Can you work these out from the model? Positions are in its coordinate system, mm. A direction names the side the tool comes from. Coordinates: 2 decimals unless noted, no trailing zeros. Order: outer loops, then holes, each group sorted by start corner. A loop starts at its lowest first (then second) coordinate and runs counter-clockwise, first axis right, second up. Notation, with made-up numbers: (-38, 51) -> (-1, 51) arc R20 ccw to (-1, 80) -> close; hole circle Ø2 at (67.5, 53). An arc over 180 degrees is marked (long way). Answer in a Markdown table with one row per item. Add a question column.
1. If I drill on line 1 along Z through (x, y) = (0.7, 23); line 2 along Y through (x, z) = (0.5, -60); line 3 along Y through (x, z) = (0.35, -26), over which ranges is the centre line in solid material (lowest first)? Write a range as [from, to].
2. Will these pins go through, and if not, where does the flat tip stop? pin 1 (1 mm diameter, centred on x = 0.5, z = -107.5, fed in from +Y); pin 2 (1 mm diameter, centred on x = 1.5, z = -105, fed in from -Y); pin 3 (1 mm diameter, centred on x = 1.5, y = 32, fed in from +Z); pin 4 (4 mm diameter, centred on y = 23.5, z = -82.5, fed in from -X).
3. We'd pull the mould along Y, two halves only. Please class faces 4 (the face through (1.01, 25.4, -6.57)), 5 (the face through (1, 16, 5)), 6 (the face through (1, 31, -2)): pulls with the +Y half, pulls with the -Y half, needs draft (parallel to the pull), parting line crosses it, or undercut.
4. Imagine slicing it at A-A on z = -78. Write out the boundary of the cut face in (x, y).
5. Imagine slicing it at D-D on x = 0.4. State how many separate pieces and enclosed holes the cut face has, plus the area to 3 significant figures.
6. Imagine slicing it at C-C on z = -45. Write out the boundary of the cut face in (x, y).
7. On a 3-axis mill with a long thin cutter (end or side, diameter ignored), from which of +Z, -Z, +X, -X, +Y, -Y can I reach the whole of each face in a straight line? I mean faces 1 (the face through (1, 18, 1)), 2 (the face through (1, 32, -82)), 3 (the face through (1, 31, -106)). Say none if no direction works.
8. Imagine slicing it at B-B on y = 6. Write out the boundary of the cut face in (x, z).
from build123d import *

# Parameters (mm, degrees)
SKETCH_1_W          = 107
SKETCH_1_H          = 31
EXTRUDE_1_DEPTH     = 2
EXTRUDE_2_DEPTH     = 2
CUT_EXTRUDE_1_DEPTH = 117.228223767
SKETCH_5_W          = 15
SKETCH_5_H          = 2.5
EXTRUDE_3_DEPTH     = 2
CUT_EXTRUDE_2_DEPTH = 117.919844338
CUT_EXTRUDE_3_DEPTH = 117.919844338


with BuildPart() as part:
    # 草图1 → 凸台-拉伸1 (new body)
    with BuildSketch(Plane(origin=(0, 0, 0), x_dir=(0, 0, -1), z_dir=(1, 0, 0))):
        with Locations((53.5, 15.5)):
            Rectangle(SKETCH_1_W, SKETCH_1_H)
    extrude(amount=EXTRUDE_1_DEPTH)

    # 草图2 → 凸台-拉伸2 (add)
    with BuildSketch(Plane(origin=(2, 0, 0), x_dir=(0, 0, -1), z_dir=(1, 0, 0))):
        Polygon((0, 31), (-5, 31), (-5, 0), (0, 0), (0, 5), (-2.1, 5), (-2.1, 13), (0, 13), (0, 18), (-2.1, 18), (-2.1, 26), (0, 26), align=None)
        Polygon((107, 0), (107, 5), (109.1, 5), (109.1, 13), (107, 13), (107, 18), (109.1, 18), (109.1, 26), (107, 26), (107, 31), (112, 31), (112, 0), align=None)
    extrude(amount=-EXTRUDE_2_DEPTH)

    # 草图3 → 切除-拉伸1 (cut, through all)
    with BuildSketch(Plane(origin=(2, 0, 0), x_dir=(0, 0, -1), z_dir=(1, 0, 0))):
        with BuildLine():
            Line((-2.1, 24), (-2.1, 26))
            ThreePointArc((-2.1, 26), (-3.1, 25), (-2.1, 24))
        make_face()
        with BuildLine():
            Line((0, 24), (0, 26))
            ThreePointArc((0, 26), (1, 25), (0, 24))
        make_face()
        with BuildLine():
            Line((0, 20), (0, 18))
            ThreePointArc((0, 18), (1, 19), (0, 20))
        make_face()
        with BuildLine():
            Line((-2.1, 20), (-2.1, 18))
            ThreePointArc((-2.1, 18), (-3.1, 19), (-2.1, 20))
        make_face()
        with BuildLine():
            Line((-2.1, 11), (-2.1, 13))
            ThreePointArc((-2.1, 13), (-3.1, 12), (-2.1, 11))
        make_face()
        with BuildLine():
            Line((0, 11), (0, 13))
            ThreePointArc((0, 13), (1, 12), (0, 11))
        make_face()
        with BuildLine():
            Line((0, 7), (0, 5))
            ThreePointArc((0, 5), (1, 6), (0, 7))
        make_face()
        with BuildLine():
            Line((-2.1, 7), (-2.1, 5))
            ThreePointArc((-2.1, 5), (-3.1, 6), (-2.1, 7))
        make_face()
        with BuildLine():
            Line((109.1, 7), (109.1, 5))
            ThreePointArc((109.1, 5), (110.1, 6), (109.1, 7))
        make_face()
        with BuildLine():
            Line((107, 7), (107, 5))
            ThreePointArc((107, 5), (106, 6), (107, 7))
        make_face()
        with BuildLine():
            Line((107, 11), (107, 13))
            ThreePointArc((107, 13), (106, 12), (107, 11))
        make_face()
        with BuildLine():
            Line((109.1, 11), (109.1, 13))
            ThreePointArc((109.1, 13), (110.1, 12), (109.1, 11))
        make_face()
        with BuildLine():
            Line((109.1, 20), (109.1, 18))
            ThreePointArc((109.1, 18), (110.1, 19), (109.1, 20))
        make_face()
        with BuildLine():
            Line((107, 20), (107, 18))
            ThreePointArc((107, 18), (106, 19), (107, 20))
        make_face()
        with BuildLine():
            Line((107, 24), (107, 26))
            ThreePointArc((107, 26), (106, 25), (107, 24))
        make_face()
        with BuildLine():
            Line((109.1, 24), (109.1, 26))
            ThreePointArc((109.1, 26), (110.1, 25), (109.1, 24))
        make_face()
    extrude(amount=-CUT_EXTRUDE_1_DEPTH, mode=Mode.SUBTRACT)

    # 草图5 → 凸台-拉伸3 (add)
    with BuildSketch(Plane(origin=(2, 0, 0), x_dir=(0, 0, -1), z_dir=(1, 0, 0))):
        with Locations((17.5, 32.25)):
            Rectangle(SKETCH_5_W, SKETCH_5_H)
        with Locations((53.5, 32.25)):
            Rectangle(SKETCH_5_W, SKETCH_5_H)
        with Locations((89.5, 32.25)):
            Rectangle(SKETCH_5_W, SKETCH_5_H)
        with Locations((89.5, -1.25)):
            Rectangle(SKETCH_5_W, SKETCH_5_H)
        with Locations((53.5, -1.25)):
            Rectangle(SKETCH_5_W, SKETCH_5_H)
        with Locations((17.5, -1.25)):
            Rectangle(SKETCH_5_W, SKETCH_5_H)
    extrude(amount=-EXTRUDE_3_DEPTH)

    # 草图6 → 切除-拉伸2 (cut, through all)
    with BuildSketch(Plane(origin=(2, 0, 0), x_dir=(0, 0, -1), z_dir=(1, 0, 0))):
        with BuildLine():
            Line((10, 31), (8, 31))
            ThreePointArc((8, 31), (9, 30), (10, 31))
        make_face()
        with BuildLine():
            Line((25, 31), (27, 31))
            ThreePointArc((27, 31), (26, 30), (25, 31))
        make_face()
        with BuildLine():
            Line((46, 31), (44, 31))
            ThreePointArc((44, 31), (45, 30), (46, 31))
        make_face()
        with BuildLine():
            Line((61, 31), (63, 31))
            ThreePointArc((63, 31), (62, 30), (61, 31))
        make_face()
        with BuildLine():
            Line((82, 31), (80, 31))
            ThreePointArc((80, 31), (81, 30), (82, 31))
        make_face()
        with BuildLine():
            Line((97, 31), (99, 31))
            ThreePointArc((99, 31), (98, 30), (97, 31))
        make_face()
        with BuildLine():
            Line((97, 0), (99, 0))
            ThreePointArc((99, 0), (98, 1), (97, 0))
        make_face()
        with BuildLine():
            Line((82, 0), (80, 0))
            ThreePointArc((80, 0), (81, 1), (82, 0))
        make_face()
        with BuildLine():
            Line((61, 0), (63, 0))
            ThreePointArc((63, 0), (62, 1), (61, 0))
        make_face()
        with BuildLine():
            Line((46, 0), (44, 0))
            ThreePointArc((44, 0), (45, 1), (46, 0))
        make_face()
        with BuildLine():
            Line((25, 0), (27, 0))
            ThreePointArc((27, 0), (26, 1), (25, 0))
        make_face()
        with BuildLine():
            Line((10, 0), (8, 0))
            ThreePointArc((8, 0), (9, 1), (10, 0))
        make_face()
    extrude(amount=-CUT_EXTRUDE_2_DEPTH, mode=Mode.SUBTRACT)

    # 草图7 → 切除-拉伸3 (cut, through all)
    with BuildSketch(Plane(origin=(2, 0, 0), x_dir=(0, 0, -1), z_dir=(1, 0, 0))):
        with BuildLine():
            Line((8, 26), (32, 26))
            ThreePointArc((32, 26), (33.414213562, 25.414213562), (34, 24))
            Line((34, 24), (34, 20))
            ThreePointArc((34, 20), (33.414213562, 18.585786438), (32, 18))
            Line((32, 18), (8, 18))
            ThreePointArc((8, 18), (6.585786438, 18.585786438), (6, 20))
            Line((6, 20), (6, 24))
            ThreePointArc((6, 24), (6.585786438, 25.414213562), (8, 26))
        make_face()
        with BuildLine():
            Line((39.5, 24), (39.5, 20))
            ThreePointArc((39.5, 20), (40.085786438, 18.585786438), (41.5, 18))
            Line((41.5, 18), (65.5, 18))
            ThreePointArc((65.5, 18), (66.914213562, 18.585786438), (67.5, 20))
            Line((67.5, 20), (67.5, 24))
            ThreePointArc((67.5, 24), (66.914213562, 25.414213562), (65.5, 26))
            Line((65.5, 26), (41.5, 26))
            ThreePointArc((41.5, 26), (40.085786438, 25.414213562), (39.5, 24))
        make_face()
        with BuildLine():
            Line((73, 24), (73, 20))
            ThreePointArc((73, 20), (73.585786438, 18.585786438), (75, 18))
            Line((75, 18), (99, 18))
            ThreePointArc((99, 18), (100.414213562, 18.585786438), (101, 20))
            Line((101, 20), (101, 24))
            ThreePointArc((101, 24), (100.414213562, 25.414213562), (99, 26))
            Line((99, 26), (75, 26))
            ThreePointArc((75, 26), (73.585786438, 25.414213562), (73, 24))
        make_face()
        with BuildLine():
            Line((39.5, 11), (39.5, 7))
            ThreePointArc((39.5, 7), (40.085786438, 5.585786438), (41.5, 5))
            Line((41.5, 5), (65.5, 5))
            ThreePointArc((65.5, 5), (66.914213562, 5.585786438), (67.5, 7))
            Line((67.5, 7), (67.5, 11))
            ThreePointArc((67.5, 11), (66.914213562, 12.414213562), (65.5, 13))
            Line((65.5, 13), (41.5, 13))
            ThreePointArc((41.5, 13), (40.085786438, 12.414213562), (39.5, 11))
        make_face()
        with BuildLine():
            Line((73, 11), (73, 7))
            ThreePointArc((73, 7), (73.585786438, 5.585786438), (75, 5))
            Line((75, 5), (99, 5))
            ThreePointArc((99, 5), (100.414213562, 5.585786438), (101, 7))
            Line((101, 7), (101, 11))
            ThreePointArc((101, 11), (100.414213562, 12.414213562), (99, 13))
            Line((99, 13), (75, 13))
            ThreePointArc((75, 13), (73.585786438, 12.414213562), (73, 11))
        make_face()
        with BuildLine():
            Line((6, 11), (6, 7))
            ThreePointArc((6, 7), (6.585786438, 5.585786438), (8, 5))
            Line((8, 5), (32, 5))
            ThreePointArc((32, 5), (33.414213562, 5.585786438), (34, 7))
            Line((34, 7), (34, 11))
            ThreePointArc((34, 11), (33.414213562, 12.414213562), (32, 13))
            Line((32, 13), (8, 13))
            ThreePointArc((8, 13), (6.585786438, 12.414213562), (6, 11))
        make_face()
    extrude(amount=-CUT_EXTRUDE_3_DEPTH, mode=Mode.SUBTRACT)


solid = part.part
Answers follow:
| question | item | result |
|---|---|---|
| 1 | line 1 | z = [-112, -109.1], [-107, -101], [-73, -67.5], [-39.5, -34], [-6, 0], [2.1, 5] |
| 1 | line 2 | y = [-2.5, 5], [13, 18], [26, 33.5] |
| 1 | line 3 | y = [1, 5], [13, 18], [26, 30] |
| 2 | pin 1 | stops at y = 31 |
| 2 | pin 2 | stops at y = 0 |
| 2 | pin 3 | stops at z = -10 |
| 2 | pin 4 | passes through |
| 3 | face 4 | undercut |
| 3 | face 5 | needs draft |
| 3 | face 6 | pulls with the +Y half |
| 4 | outline | (0, 0) -> (2, 0) -> (2, 5) -> (0, 5) -> close; (0, 13) -> (2, 13) -> (2, 18) -> (0, 18) -> close; (0, 26) -> (2, 26) -> (2, 31) -> (0, 31) -> close |
| 5 | separate pieces | 1 |
| 5 | enclosed holes | 10 |
| 5 | area | 2,420 mm² |
| 6 | outline | (0, 1) -> (2, 1) -> (2, 5) -> (0, 5) -> close; (0, 13) -> (2, 13) -> (2, 18) -> (0, 18) -> close; (0, 26) -> (2, 26) -> (2, 30) -> (0, 30) -> close |
| 7 | face 1 | +X, -X |
| 7 | face 2 | +X, -X, +Y |
| 7 | face 3 | -Z, +X, -X, +Y |
| 8 | outline | (0, -112) -> (2, -112) -> (2, -110.1) -> (0, -110.1) -> close; (0, -106) -> (2, -106) -> (2, -100.73) -> (0, -100.73) -> close; (0, -73.27) -> (2, -73.27) -> (2, -67.23) -> (0, -67.23) -> close; (0, -39.77) -> (2, -39.77) -> (2, -33.73) -> (0, -33.73) -> close; (0, -6.27) -> (2, -6.27) -> (2, -1) -> (0, -1) -> close; (0, 3.1) -> (2, 3.1) -> (2, 5) -> (0, 5) -> close |
